from build123d import *

# Parameters (mm, degrees)
SKETCH_2_W             = 40
SKETCH_2_H             = 23
SKETCH_2_R             = 1
EXTRUDE_1815_DEPTH     = 5
SKETCH_3_W             = 37
SKETCH_3_H             = 20
CUT_EXTRUDE_2215_DEPTH = 3
SKETCH_4_R             = 1
EXTRUDE_2889_DEPTH     = 1.9
SKETCH_10_R            = 0.5
EXTRUDE_4733_DEPTH     = 5
FILLET_START           = -1
FILLET_5_DEPTH         = 7
FILLET_6_DEPTH         = 7
CUT_EXTRUDE_7304_DEPTH = 1.1


with BuildPart() as part:
    # Эскиз2 → Extrude 1815 (new body)
    with BuildSketch(Plane.XY):
        Rectangle(SKETCH_2_W, SKETCH_2_H)
        with Locations((15.7, -7.7)):
            Circle(SKETCH_2_R, mode=Mode.SUBTRACT)
        with Locations((-15.7, 7.7)):
            Circle(SKETCH_2_R, mode=Mode.SUBTRACT)
        with Locations((15.7, 7.7)):
            Circle(SKETCH_2_R, mode=Mode.SUBTRACT)
        with Locations((-15.7, -7.7)):
            Circle(SKETCH_2_R, mode=Mode.SUBTRACT)
    extrude(amount=EXTRUDE_1815_DEPTH)

    # Эскиз3 → Cut-Extrude 2215 (cut)
    with BuildSketch(Plane.XY.offset(5)):
        Rectangle(SKETCH_3_W, SKETCH_3_H)
    extrude(amount=-CUT_EXTRUDE_2215_DEPTH, mode=Mode.SUBTRACT)

    # Эскиз4 → Extrude 2889 (add)
    with BuildSketch(Plane.XY.offset(2)):
        with BuildLine():
            ThreePointArc((-17.296871942, 10), (-18.181052341, 8.997836384), (-18.5, 7.7))
            Line((-18.5, 7.7), (-18.5, -10))
            Line((-18.5, -10), (18.5, -10))
            Line((18.5, -10), (18.5, 10))
            Line((18.5, 10), (-17.296871942, 10))
        make_face()
        with Locations((-15.7, 7.7)):
            Circle(SKETCH_4_R, mode=Mode.SUBTRACT)
        with Locations((15.7, -7.7)):
            Circle(SKETCH_4_R, mode=Mode.SUBTRACT)
        with Locations((15.7, 7.7)):
            Circle(SKETCH_4_R, mode=Mode.SUBTRACT)
        with Locations((-15.7, -7.7)):
            Circle(SKETCH_4_R, mode=Mode.SUBTRACT)
    extrude(amount=EXTRUDE_2889_DEPTH)

    # Эскиз10 → Extrude 4733 (add)
    # profile 1 of 4: a face of its own
    with BuildSketch(Plane(origin=(0, 0, 0), x_dir=(-1, 0, 0), z_dir=(0, 0, -1))):
        with BuildLine():
            Line((-17.5, 14), (-17.5, 13.5))
            ThreePointArc((-17.5, 13.5), (-18.085786438, 12.085786438), (-19.5, 11.5))
            Line((-19.5, 11.5), (-10.5, 11.5))
            ThreePointArc((-10.5, 11.5), (-11.914213562, 12.085786438), (-12.5, 13.5))
            Line((-12.5, 13.5), (-12.5, 14))
            ThreePointArc((-12.5, 14), (-15, 16.5), (-17.5, 14))
        make_face()
        with Locations((-15, 14)):
            Circle(SKETCH_10_R, mode=Mode.SUBTRACT)
    # profile 2 of 4: a face of its own
    with BuildSketch(Plane(origin=(0, 0, 0), x_dir=(-1, 0, 0), z_dir=(0, 0, -1))):
        with BuildLine():
            Line((10.5, 11.5), (19.5, 11.5))
            ThreePointArc((19.5, 11.5), (18.085786438, 12.085786438), (17.5, 13.5))
            Line((17.5, 13.5), (17.5, 14))
            ThreePointArc((17.5, 14), (15, 16.5), (12.5, 14))
            Line((12.5, 14), (12.5, 13.5))
            ThreePointArc((12.5, 13.5), (11.914213562, 12.085786438), (10.5, 11.5))
        make_face()
        with Locations(Location((15, 14, 0), (0, 0, 180))):
            Circle(SKETCH_10_R, mode=Mode.SUBTRACT)
    # profile 3 of 4: a face of its own
    with BuildSketch(Plane(origin=(0, 0, 0), x_dir=(-1, 0, 0), z_dir=(0, 0, -1))):
        with BuildLine():
            Line((17.5, -14), (17.5, -13.5))
            ThreePointArc((17.5, -13.5), (18.085786438, -12.085786438), (19.5, -11.5))
            Line((19.5, -11.5), (10.5, -11.5))
            ThreePointArc((10.5, -11.5), (11.914213562, -12.085786438), (12.5, -13.5))
            Line((12.5, -13.5), (12.5, -14))
            ThreePointArc((12.5, -14), (15, -16.5), (17.5, -14))
        make_face()
        with Locations((15, -14)):
            Circle(SKETCH_10_R, mode=Mode.SUBTRACT)
    # profile 4 of 4: a face of its own
    with BuildSketch(Plane(origin=(0, 0, 0), x_dir=(-1, 0, 0), z_dir=(0, 0, -1))):
        with BuildLine():
            Line((-10.5, -11.5), (-19.5, -11.5))
            ThreePointArc((-19.5, -11.5), (-18.085786438, -12.085786438), (-17.5, -13.5))
            Line((-17.5, -13.5), (-17.5, -14))
            ThreePointArc((-17.5, -14), (-15, -16.5), (-12.5, -14))
            Line((-12.5, -14), (-12.5, -13.5))
            ThreePointArc((-12.5, -13.5), (-11.914213562, -12.085786438), (-10.5, -11.5))
        make_face()
        with Locations(Location((-15, -14, 0), (0, 0, 180))):
            Circle(SKETCH_10_R, mode=Mode.SUBTRACT)
    extrude(amount=-EXTRUDE_4733_DEPTH)

    # Скругление5: read off the stored shape, not the designer's step
    # Скругление5 outline → Скругление5 (cut)
    with BuildSketch(Plane.XY.offset(FILLET_START)):
        with BuildLine():
            ThreePointArc((19.5, 11.5), (18.5867215, 11.720696097), (17.875, 12.334077619))
            add(Edge.make_bspline(
                [(17.875, 12.334077619), (20, 9.372366741), (20, 8.836310473)],
                knots=[0, 0, 0, 1, 1, 1], degree=2, weights=[1, 1.5, 1]))
            Line((20, 8.836310473), (20, 11.5))
            Line((20, 11.5), (19.5, 11.5))
        make_face()
        with BuildLine():
            ThreePointArc((-19.5, -11.5), (-18.5867215, -11.720696097), (-17.875, -12.334077619))
            add(Edge.make_bspline(
                [(-17.875, -12.334077619), (-20, -9.372366741), (-20, -8.836310473)],
                knots=[0, 0, 0, 1, 1, 1], degree=2, weights=[1, 1.5, 1]))
            Line((-20, -8.836310473), (-20, -11.5))
            Line((-20, -11.5), (-19.5, -11.5))
        make_face()
    extrude(amount=FILLET_5_DEPTH, mode=Mode.SUBTRACT)

    # Скругление6: read off the stored shape, not the designer's step
    # Скругление6 outline → Скругление6 (cut)
    with BuildSketch(Plane.XY.offset(FILLET_START)):
        with BuildLine():
            add(Edge.make_bspline(
                [(-17.875, 12.334077618), (-20, 9.372366741), (-20, 8.836310473)],
                knots=[0, 0, 0, 1, 1, 1], degree=2, weights=[1, 1.5, 1]))
            ThreePointArc((-17.875, 12.334077618), (-18.5867215, 11.720696097), (-19.5, 11.5))
            Line((-19.5, 11.5), (-20, 11.5))
            Line((-20, 11.5), (-20, 8.836310473))
        make_face()
        with BuildLine():
            add(Edge.make_bspline(
                [(17.875, -12.334077618), (20, -9.372366741), (20, -8.836310473)],
                knots=[0, 0, 0, 1, 1, 1], degree=2, weights=[1, 1.5, 1]))
            ThreePointArc((17.875, -12.334077618), (18.5867215, -11.720696097), (19.5, -11.5))
            Line((19.5, -11.5), (20, -11.5))
            Line((20, -11.5), (20, -8.836310473))
        make_face()
    extrude(amount=FILLET_6_DEPTH, mode=Mode.SUBTRACT)

    # Эскиз12 → Cut-Extrude 7304 (cut)
    with BuildSketch(Plane.XY.offset(5)):
        with BuildLine():
            Line((-5.593541674, 13.75), (-10.5, 13.75))
            ThreePointArc((-10.5, 13.75), (-11.076220456, 13.834805496), (-11.60357425, 14.082030014))
            ThreePointArc((-11.60357425, 14.082030014), (-8.693066451, 12.205329008), (-5.593541674, 13.75))
        make_face()
        with BuildLine():
            Line((3.993541674, -13.75), (9.806458326, -13.75))
            ThreePointArc((9.806458326, -13.75), (6.9, -12.2), (3.993541674, -13.75))
        make_face()
    extrude(amount=-CUT_EXTRUDE_7304_DEPTH, mode=Mode.SUBTRACT)


solid = part.part
Input: part model. Units: mm. Frame: model coordinates. A direction names the side the tool comes from. Round coordinates to 2 decimals unless told otherwise and drop trailing zeros. Loops run counter-clockwise (first coordinate to the right, second up) from the corner with the lowest first, then second, coordinate; pieces in that order, holes last. Notation, with made-up numbers: (83, -8.75) -> (135, -8.75) arc R17 cw to (135, -1.75) -> close; hole circle Ø9 at (76, 70.5). An arc over 180 degrees is marked (long way). Answer as a JSON object with one key per item and string values. Group by question number.
1) Section query D-D on x = 13. Output: boundary loops of the cut face in (y, z), plus the area to 3 significant figures.
2) Reachability of faces 5 (the cylindrical face through (-11.93, 12.1, 2.46)), 6 (the cylindrical face through (-17.6, 12.88, 2.46)), 7 (the flat face through (18.5, -0.1, 4.5)) from +Z, -Z, +X, -X, +Y, -Y: full face, straight path, thin tool, end or side. Return the list, or none.
3) Ray query, L1, parallel to Y at x = 15, z = 3; L2, parallel to Y at x = -15.7, z = 3.15; L3, parallel to Z at x = 2, y = -1.5. Return the intervals inside material, ascending.
4) Pin query (flat end, axial travel): pin 1 (0.6 mm diameter, centred on x = -4, z = 4.5, fed in from +Y); pin 2 (0.6 mm diameter, centred on y = -13.5, z = 3, fed in from +X); pin 3 (2.5 mm diameter, centred on x = 9, z = 3.5, fed in from -Y). Return the tip coordinate at first contact, or that it passes through.
5) Section query C-C on z = 3.1. State how many separate pieces and enclosed holes the cut face has, plus the area to 3 significant figures.
6) Section query A-A on y = -7.7. Output: boundary loops of the cut face in (x, z), plus the area to 3 significant figures.
7) Draft query along Y for faces 1 (the cylindrical face through (11.9, 12.07, 2.46)), 2 (the flat face through (0, -11.5, 2)), 3 (the flat face through (-18.1, 9.5, 2)), 4 (the flat face through (-20, 0, 2)). Return one class per face: +Y half, -Y half, draft (parallel to the pull), parting line (faces both ways), or undercut.
8) Section query B-B on x = -2. Output: boundary loops of the cut face in (y, z), plus the area to 3 significant figures.
Reply:
{
 "1": {"outline": "(-15.5, 0) -> (15.5, 0) -> (15.5, 5) -> (10, 5) -> (10, 3.9) -> (-10, 3.9) -> (-10, 5) -> (-15.5, 5) -> close", "area": "133 mm2"},
 "2": {"face 5": "+Z, -Z, +Y", "face 6": "+Z, -Z, -X, +Y", "face 7": "+Z"},
 "3": {"L1": "y = -16.5 to -14.5, -13.5 to -8.41, -6.99 to 6.99, 8.41 to 13.5, 14.5 to 16.5", "L2": "y = -16.4 to -8.7, -6.7 to 6.7, 8.7 to 16.4", "L3": "z = 0 to 3.9"},
 "4": {"pin 1": "stops at y = 11.5", "pin 2": "stops at x = 17.52", "pin 3": "stops at y = -11.5"},
 "5": {"separate pieces": "1", "enclosed holes": "9", "area": "992 mm2"},
 "6": {"outline": "(-20, 0) -> (-16.7, 0) -> (-16.7, 3.9) -> (-18.5, 3.9) -> (-18.5, 5) -> (-20, 5) -> close; (-14.7, 0) -> (14.7, 0) -> (14.7, 3.9) -> (-14.7, 3.9) -> close; (16.7, 0) -> (20, 0) -> (20, 5) -> (18.5, 5) -> (18.5, 3.9) -> (16.7, 3.9) -> close", "area": "144 mm2"},
 "7": {"face 1": "+Y half", "face 2": "-Y half", "face 3": "undercut", "face 4": "draft"},
 "8": {"outline": "(-11.5, 0) -> (11.5, 0) -> (11.5, 5) -> (10, 5) -> (10, 3.9) -> (-10, 3.9) -> (-10, 5) -> (-11.5, 5) -> close", "area": "93.0 mm2"}
}
